Geometry: final body of the model. Coordinates: model frame, mm. A direction names the side the tool comes from. Give positions to 0.01 mm unless a question says otherwise; leave off trailing zeros. Write each loop counter-clockwise with the first axis right and the second up, starting at its lowest first coordinate (ties: lowest second). Pieces come first, ordered by that corner, then holes. Notation, with made-up numbers: M 78,4 L 123,4 A17 ccw 123,19 Z; hole C 4.25,87 d8. An arc over 180 degrees is marked long. Use a Markdown table: item, result. Add a question column.
(1) Reachability of faces 1 (the flat face through (-1, 0, 1)), 2 (the flat face through (172.72, 361, 38)) from +Z, -Z, +X, -X, +Y, -Y: full face, straight path, thin tool, end or side. Return the list, or none.
(2) Draft query along X for faces 3 (the flat face through (-172.72, 361, 37)), 4 (the flat face through (-2, 363, 0)), 5 (the flat face through (177.8, 363, 34)), 6 (the flat face through (-177.8, 363, 35)). Return one class per face: released by +X, released by -X, zero draft, split by the parting line, or undercut.
(3) Material intervals for L1, parallel to X at y = 399, z = 55; L2, parallel to Y at x = -47.5, z = 32; L3, parallel to Z at x = -111, y = 151, sorted ascending.
(4) Cut plane A-A (y = 97.5). Output: boundary loops of the cut face in (x, z).
(5) Cut plane C-C (x = -84). Output: boundary loops of the cut face in (y, z), plus the area to 3 significant figures.
(6) Pin query (flat end, axial travel): pin 1 Ø12 at (x, z) = (2, 48.5) entering from -Y. Return the tip coordinate at first contact, or that it passes through.
(7) Cut plane B-B (z = 30). Output: boundary loops of the cut face in (x, y).
```python
from build123d import *

# Parameters (mm, degrees)
F1_DEPTH = 736.6
F2_W     = 345.44
F2_H     = 5.08
F3_DEPTH = 64.77


with BuildPart() as f1:
    # F0 (on Front) → F1 (new body)
    with BuildSketch(Plane.XZ):
        Polygon((-172.72, 69.85), (-177.8, 69.85), (-177.8, 0), (177.8, 0), (177.8, 69.85), (172.72, 69.85), (172.72, 5.08), (-172.72, 5.08), align=None)
    extrude(amount=-F1_DEPTH)

    # F2 (on face) → F3 (join, through all)
    with BuildSketch(Plane.XY.offset(5.08)):
        with Locations((0, 734.06)):
            Rectangle(F2_W, F2_H)
    extrude(amount=F3_DEPTH)


solid = f1.part
```
Answer list:
| question | item | result |
|---|---|---|
| 1 | face 1 | +Z, -Z, +X, -X, -Y |
| 1 | face 2 | +Z, -Y |
| 2 | face 3 | undercut |
| 2 | face 4 | zero draft |
| 2 | face 5 | released by +X |
| 2 | face 6 | released by -X |
| 3 | L1 | -177.8 to -172.72, 172.72 to 177.8 |
| 3 | L2 | 731.52 to 736.6 |
| 3 | L3 | 0 to 5.08 |
| 4 | outline | M -177.8,0 L 177.8,0 L 177.8,69.85 L 172.72,69.85 L 172.72,5.08 L -172.72,5.08 L -172.72,69.85 L -177.8,69.85 Z |
| 5 | outline | M 0,0 L 736.6,0 L 736.6,69.85 L 731.52,69.85 L 731.52,5.08 L 0,5.08 Z |
| 5 | area | 4,070 mm² |
| 6 | pin 1 | y = 731.52 |
| 7 | outline | M -177.8,0 L -172.72,0 L -172.72,731.52 L 172.72,731.52 L 172.72,0 L 177.8,0 L 177.8,736.6 L -177.8,736.6 Z |
